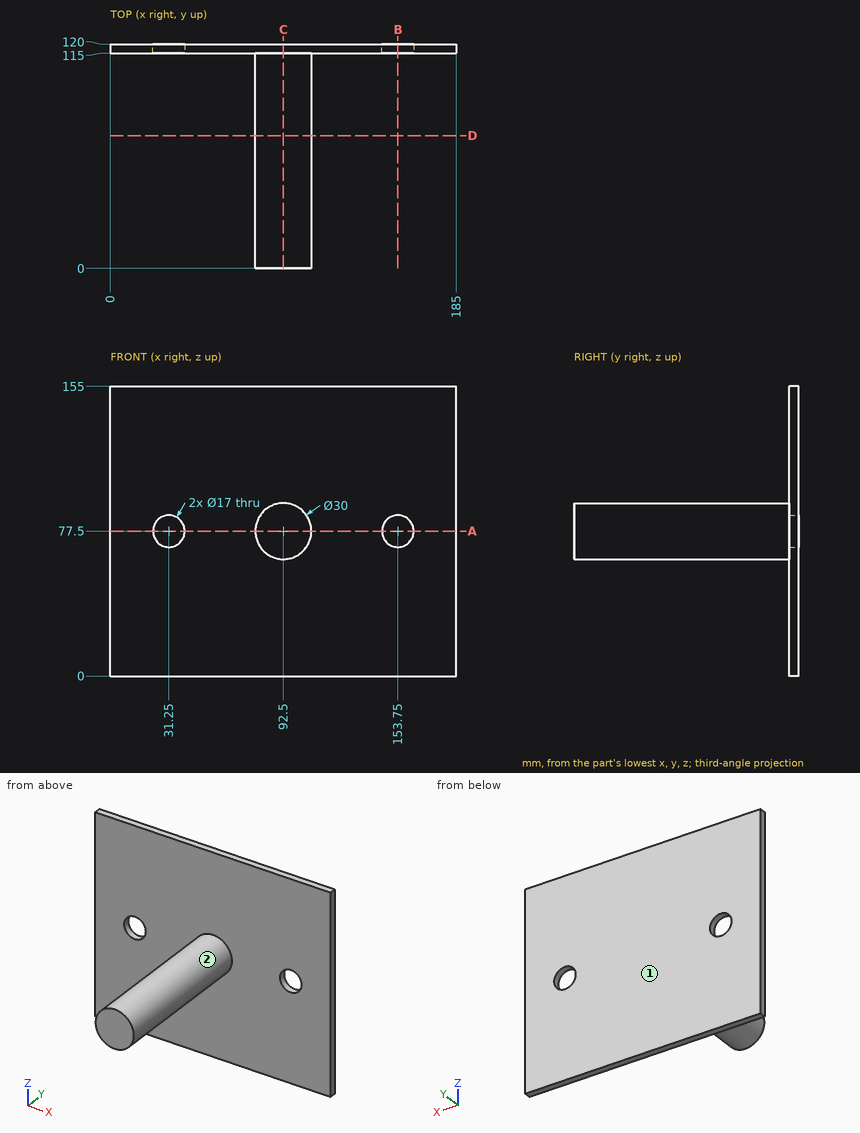
The figure shows three views and two pictorial views of one solid part (mm, origin at its lowest corner). Answer the questions. A direction names the side the tool comes from. Give positions to 0.01 mm unless a question says otherwise; leave off trailing zeros. Loops run counter-clockwise (first coordinate to the right, second up) from the corner with the lowest first, then second, coordinate; pieces in that order, holes last. Notation, with made-up numbers: (-32.5, 67) - (4.5, 67) arc R10 ccw to (4.5, 75) - close; hole circle Ø3 at (65, 33.5). An arc over 180 degrees is marked (long way). Use one line per item in the form item = value.
1. Given pin 1 Ø13.5 at (x, z) = (31.25, 77.5) entering from +Y; pin 2 Ø1 at (x, z) = (69, 36.5) entering from -Y, each flat-ended and moving along its own axis, determine where each tip first touches the part or whether it passes through.
Calculated:
pin_1 = through
pin_2 = 115
2. Find the intervals of material crossed by line 1 along X through (y, z) = (118, 77); line 2 along Z through (x, y) = (31, 117); line 3 along Y through (x, z) = (119.5, 22), in increasing order. Write a range as [from, to].
Calculated:
line_1 = [0, 22.76], [39.74, 145.26], [162.24, 185]
line_2 = [0, 69], [86, 155]
line_3 = [115, 120]
3. Section D-D on y = 71 is taken. Give the vertices of the cut face in (x, z), then the cut area to 3 significant figures.
Calculated:
outline = circle Ø30 at (92.5, 77.5)
area = 707 mm^2
4. Section B-B on x = 153.75 is taken. Give the vertices of the cut face in (y, z), then the cut area to 3 significant figures.
Calculated:
outline = (115, 0) - (120, 0) - (120, 69) - (115, 69) - close; (115, 86) - (120, 86) - (120, 155) - (115, 155) - close
area = 690 mm^2
5. Section A-A on z = 77.5 is taken. Give the vertices of the cut face in (x, y), then the cut area to 4 significant figures.
Calculated:
outline = (0, 115) - (22.75, 115) - (22.75, 120) - (0, 120) - close; (39.75, 115) - (77.5, 115) - (77.5, 0) - (107.5, 0) - (107.5, 115) - (145.25, 115) - (145.25, 120) - (39.75, 120) - close; (162.25, 115) - (185, 115) - (185, 120) - (162.25, 120) - close
area = 4,205 mm^2
6. Which of the six approach directions +Z, -Z, +X, -X, +Y, -Y give full straight-line access (tool end or side, diameter ignored) to the marked faces 1 and 2?
Calculated:
face_1 = +Z, -Z, +X, -X, +Y
face_2 = -Y
7. Section C-C on x = 92.5 is taken. Give the vertices of the cut face in (y, z), then the cut area to 4 significant figures.
Calculated:
outline = (0, 62.5) - (115, 62.5) - (115, 0) - (120, 0) - (120, 155) - (115, 155) - (115, 92.5) - (0, 92.5) - close
area = 4,225 mm^2
